Work out the finished part from the listing and answer in its coordinate system (mm). A direction names the side the tool comes from. Give positions to 0.01 mm unless a question says otherwise; leave off trailing zeros. Loops run counter-clockwise (first coordinate to the right, second up) from the corner with the lowest first, then second, coordinate; pieces in that order, holes last. Notation, with made-up numbers: (-39, 67.5) - (-20, 67.5) arc R30 cw to (-20, 89.5) - close; hole circle Ø7 at (62, 4.5). An arc over 180 degrees is marked (long way). One line per question, with ' | ' between items. Start each with the question number.
1. Which of the six approach directions +Z, -Z, +X, -X, +Y, -Y give full straight-line access (tool end or side, diameter ignored) to faces 1 (the face through (10.916, 49.094, 35.636)), 2 (the face through (0.773, 24.715, 38.765)), 3 (the face through (58.227, -22.278, 20.428))?
2. Find the intervals of material crossed by line 1 (Y direction, x = 12, z = -1); line 2 (Y direction, x = 10.5, z = 9.5); line 3 (Z direction, x = 16.5, y = -2), in increasing order.
3. For a pull along Z with two mould halves and no side action, classify faces 4 (the face through (20.574, -18, -35)), 5 (the face through (10.916, 35.636, -49.094)), 6 (the face through (11.182, -60.47, -46.367)) as released by +Z, released by -Z, zero draft, split by the parting line, or undercut.
4. Each of these flat-tipped pins is pushed along its axis until it touches: pin 1 (15 mm diameter, centred on y = 42.66, z = 42.66, fed in from -X); pin 2 (22 mm diameter, centred on y = 42.66, z = -42.66, fed in from -X); pin 3 (6 mm diameter, centred on y = -28, z = -57, fed in from +X); pin 4 (3 mm diameter, centred on x = 7, y = 22.5, fed in from +Z). Where does it stop, or does it pass through?
5. Section A-A (z = 0) is taken. Determine the outline of the cut face in (x, y), plus the area to 3 significant figures.
6. Section C-C (x = 34.5) is taken. Determine the outline of the cut face in (y, z).
7. Section D-D (z = -36) is taken. Give the number of separate pieces and of enclosed holes in the cut face, plus the area to 3 significant figures.
Autodesk Inventor part; units mm, degrees
ref_plane "YZ Plane" through (0, 0, 0) normal (1, 0, 0) x (0, 1, 0)
ref_plane "XZ Plane" through (0, 0, 0) normal (0, 1, 0) x (-1, 0, 0)
ref_plane "XY Plane" through (0, 0, 0) normal (0, 0, 1) x (1, 0, 0)
sketch "Sketch1" plane through (0, 0, 0) normal (0, 0, 1) x (1, 0, 0)
  line L0 (0, 0) -> (0, 45.974)
  line L1 (0, 45.974) -> (1.524, 45.974)
  line L2 (1.524, 45.974) -> (1.524, 76.2)
  line L3 (1.524, 76.2) -> (20.574, 76.2)
  line L4 (20.574, 76.2) -> (20.574, 38.862)
  line L5 (20.574, 38.862) -> (52.804, 30.226)
  line L6 (52.804, 30.226) -> (63.5, 30.226)
  line L7 (63.5, 30.226) -> (63.5, 0)
  line L8 (63.5, 0) -> (0, 0)
  line L9 (63.5, 26.289) -> (0, 26.289)
  dimension "d0" = 152.4
  dimension "d1" = 91.948
  dimension "d2" = 1.524
  dimension "d3" = 52.578
  dimension "d4" = 60.452
  dimension "d7" = 77.724
  dimension "d8" = 15
  dimension "d18" = 19.05
  dimension "d19" = 61.976
revolve "Revolution1" add sketch "Sketch1" angle 360 about axis through (63.5, 0, 0) along (-1, 0, 0) contours L0 L1 L2 L3 L4 L5 L6 L7 L9
sketch "Sketch2" plane through (1.524, 0, 0) normal (-1, 0, 0) x (0, 0, 1)
  circle A0 centre (0, 0) radius 76.2
  circle A1 centre (0, 0) radius 45.974
  circle A2 centre (42.6562, 42.6562) radius 9.525
  line L0 (42.6562, 42.6562) -> (0, 0) construction
  circle A3 centre (0, 0) radius 60.325 construction
  line L1 (0, 0) -> (60.325, 0) construction
  dimension "d10" = 60.325
  dimension "d11" = 19.05
  dimension "d17" = 45
extrude "Extrusion1" cut sketch "Sketch2" against normal through all contours A2
pattern_circular "Circular Pattern1" count 4 over 360 about axis through (36.689, 0, 0) along (1, 0, 0) of "Extrusion1"
equation "\"d0\" = O"
equation "\"d1\" = R"
equation "\"d3\" = B"
equation "\"d4\" = A"
equation "\"d7\" = X"
equation "\"d18\" = C1"
equation "\"d19\" = Y"
equation "\"d10\" = 0.5 * BC"
equation "\"d11\" = DH"
equation "\"O\" = 152.4"
equation "\"C1\" = 19.05"
equation "\"X\" = 77.724"
equation "\"A\" = 60.452"
equation "\"Y\" = 61.976"
equation "\"B\" = 52.578"
equation "\"BC\" = 120.65"
equation "\"DH\" = 19.05"
equation "\"R\" = 91.948"
properties part number "ASME B16.5 Flange Welding Neck - Class 150 2" material "Steel"
Conclusion:
1) face 1: +X, -X | face 2: -X | face 3: +X
2) line 1: -76.19 to -26.27, 26.27 to 76.19 | line 2: -75.61 to -24.51, 24.51 to 75.61 | line 3: -76.17 to -26.21, 26.21 to 76.17
3) face 4: zero draft | face 5: undercut | face 6: split by the parting line
4) pin 1: through | pin 2: x = 1.52 | pin 3: x = 20.57 | pin 4: z = 73.25
5) outline: (0, -45.97) - (1.52, -45.97) - (1.52, -76.2) - (20.57, -76.2) - (20.57, -38.86) - (52.8, -30.23) - (63.5, -30.23) - (63.5, -26.29) - (0, -26.29) - close; (0, 26.29) - (63.5, 26.29) - (63.5, 30.23) - (52.8, 30.23) - (20.57, 38.86) - (20.57, 76.2) - (1.52, 76.2) - (1.52, 45.97) - (0, 45.97) - close | area: 2,580 mm²
6) outline: circle Ø70.26 at (0, 0); hole circle Ø52.58 at (0, 0)
7) separate pieces: 3 | enclosed holes: 0 | area: 2,330 mm²
